```python
from build123d import *

# Parameters (mm, degrees)
SKETCH1_W           = 38.1
SKETCH1_H           = 38.1
BOSS_EXTRUDE1_DEPTH = 1.5875
SKETCH4_R           = 1.143
CUT_EXTRUDE2_DEPTH  = 7.874
SKETCH6_W           = 15.875
SKETCH6_H           = 15.875
BOSS_EXTRUDE2_DEPTH = 6.731
SKETCH7_R           = 0.889
BOSS_EXTRUDE3_DEPTH = 6.731
SKETCH8_R           = 7.747
BOSS_EXTRUDE4_DEPTH = 3.048
SKETCH9_R           = 5.969
BOSS_EXTRUDE5_DEPTH = 6.096
SKETCH10_R          = 6.985
BOSS_EXTRUDE6_DEPTH = 3.81
SKETCH11_W          = 9.906
SKETCH11_H          = 4.572
BOSS_EXTRUDE7_DEPTH = 8.255


with BuildPart() as part:
    # Sketch1 → Boss-Extrude1 (new body)
    with BuildSketch(Plane(origin=(0, 0, 0), x_dir=(1, 0, 0), z_dir=(0, 1, 0))):
        with Locations((-252.591789549, -315.673153846)):
            Rectangle(SKETCH1_W, SKETCH1_H)
    extrude(amount=BOSS_EXTRUDE1_DEPTH)

    # Sketch4 → Cut-Extrude2 (cut)
    with BuildSketch(Plane(origin=(0, 1.5875, 0), x_dir=(1, 0, 0), z_dir=(0, 1, 0))):
        with Locations((-266.561789549, -301.703153846)):
            Circle(SKETCH4_R)
        with Locations((-238.621789549, -301.703153846)):
            Circle(SKETCH4_R)
        with Locations((-266.561789549, -329.643153846)):
            Circle(SKETCH4_R)
        with Locations((-238.621789549, -329.643153846)):
            Circle(SKETCH4_R)
        with BuildLine():
            Line((-269.863789549, -312.294953846), (-269.863789549, -319.051353846))
            ThreePointArc((-269.863789549, -319.051353846), (-269.228789549, -319.686353846), (-268.593789549, -319.051353846))
            Line((-268.593789549, -319.051353846), (-268.593789549, -312.294953846))
            ThreePointArc((-268.593789549, -312.294953846), (-269.228789549, -311.659953846), (-269.863789549, -312.294953846))
        make_face()
        with BuildLine():
            Line((-259.385291519, -298.401153846), (-268.278408573, -298.401153846))
            ThreePointArc((-268.278408573, -298.401153846), (-270.0370126, -298.227930795), (-269.863789549, -299.986534822))
            Line((-269.863789549, -299.986534822), (-269.863789549, -309.246953846))
            ThreePointArc((-269.863789549, -309.246953846), (-269.228789549, -309.881953846), (-268.593789549, -309.246953846))
            Line((-268.593789549, -309.246953846), (-268.593789549, -299.986534822))
            ThreePointArc((-268.593789549, -299.986534822), (-268.420566498, -299.844376897), (-268.278408573, -299.671153846))
            Line((-268.278408573, -299.671153846), (-259.385291519, -299.671153846))
            ThreePointArc((-259.385291519, -299.671153846), (-258.750291519, -299.036153846), (-259.385291519, -298.401153846))
        make_face()
        with BuildLine():
            Line((-255.969989549, -298.401153846), (-249.213589549, -298.401153846))
            ThreePointArc((-249.213589549, -298.401153846), (-248.578589549, -299.036153846), (-249.213589549, -299.671153846))
            Line((-249.213589549, -299.671153846), (-255.969989549, -299.671153846))
            ThreePointArc((-255.969989549, -299.671153846), (-256.604989549, -299.036153846), (-255.969989549, -298.401153846))
        make_face()
        with BuildLine():
            Line((-236.589789549, -309.246953846), (-236.589789549, -299.986534822))
            ThreePointArc((-236.589789549, -299.986534822), (-236.7630126, -299.844376897), (-236.905170525, -299.671153846))
            Line((-236.905170525, -299.671153846), (-245.798287579, -299.671153846))
            ThreePointArc((-245.798287579, -299.671153846), (-246.433287579, -299.036153846), (-245.798287579, -298.401153846))
            Line((-245.798287579, -298.401153846), (-236.905170525, -298.401153846))
            ThreePointArc((-236.905170525, -298.401153846), (-235.146566498, -298.227930795), (-235.319789549, -299.986534822))
            Line((-235.319789549, -299.986534822), (-235.319789549, -309.246953846))
            ThreePointArc((-235.319789549, -309.246953846), (-235.954789549, -309.881953846), (-236.589789549, -309.246953846))
        make_face()
        with BuildLine():
            Line((-236.589789549, -312.294953846), (-236.589789549, -319.051353846))
            ThreePointArc((-236.589789549, -319.051353846), (-235.954789549, -319.686353846), (-235.319789549, -319.051353846))
            Line((-235.319789549, -319.051353846), (-235.319789549, -312.294953846))
            ThreePointArc((-235.319789549, -312.294953846), (-235.954789549, -311.659953846), (-236.589789549, -312.294953846))
        make_face()
        with BuildLine():
            Line((-245.798287579, -332.945153846), (-236.905170525, -332.945153846))
            ThreePointArc((-236.905170525, -332.945153846), (-235.146566498, -333.118376897), (-235.319789549, -331.35977287))
            Line((-235.319789549, -331.35977287), (-235.319789549, -322.099353846))
            ThreePointArc((-235.319789549, -322.099353846), (-235.954789549, -321.464353846), (-236.589789549, -322.099353846))
            Line((-236.589789549, -322.099353846), (-236.589789549, -331.35977287))
            ThreePointArc((-236.589789549, -331.35977287), (-236.7630126, -331.501930795), (-236.905170525, -331.675153846))
            Line((-236.905170525, -331.675153846), (-245.798287579, -331.675153846))
            ThreePointArc((-245.798287579, -331.675153846), (-246.433287579, -332.310153846), (-245.798287579, -332.945153846))
        make_face()
        with BuildLine():
            Line((-268.593789549, -322.099353846), (-268.593789549, -331.35977287))
            ThreePointArc((-268.593789549, -331.35977287), (-268.420566498, -331.501930795), (-268.278408573, -331.675153846))
            Line((-268.278408573, -331.675153846), (-259.385291519, -331.675153846))
            ThreePointArc((-259.385291519, -331.675153846), (-258.750291519, -332.310153846), (-259.385291519, -332.945153846))
            Line((-259.385291519, -332.945153846), (-268.278408573, -332.945153846))
            ThreePointArc((-268.278408573, -332.945153846), (-270.0370126, -333.118376897), (-269.863789549, -331.35977287))
            Line((-269.863789549, -331.35977287), (-269.863789549, -322.099353846))
            ThreePointArc((-269.863789549, -322.099353846), (-269.228789549, -321.464353846), (-268.593789549, -322.099353846))
        make_face()
        with BuildLine():
            Line((-255.969989549, -331.675153846), (-249.213589549, -331.675153846))
            ThreePointArc((-249.213589549, -331.675153846), (-248.578589549, -332.310153846), (-249.213589549, -332.945153846))
            Line((-249.213589549, -332.945153846), (-255.969989549, -332.945153846))
            ThreePointArc((-255.969989549, -332.945153846), (-256.604989549, -332.310153846), (-255.969989549, -331.675153846))
        make_face()
    extrude(amount=-CUT_EXTRUDE2_DEPTH, mode=Mode.SUBTRACT)

    # Sketch6 → Boss-Extrude2 (add)
    with BuildSketch(Plane(origin=(0, 1.5875, 0), x_dir=(1, 0, 0), z_dir=(0, 1, 0))):
        with Locations((-252.591789549, -315.673153846)):
            Rectangle(SKETCH6_W, SKETCH6_H)
    extrude(amount=BOSS_EXTRUDE2_DEPTH)

    # Sketch7 → Boss-Extrude3 (add)
    with BuildSketch(Plane(origin=(0, 1.5875, 0), x_dir=(1, 0, 0), z_dir=(0, 1, 0))):
        with BuildLine():
            Line((-242.622289549, -313.641153846), (-244.654289549, -313.641153846))
            Line((-244.654289549, -313.641153846), (-244.654289549, -317.705153846))
            Line((-244.654289549, -317.705153846), (-242.622289549, -317.705153846))
            ThreePointArc((-242.622289549, -317.705153846), (-240.590289549, -315.673153846), (-242.622289549, -313.641153846))
        make_face()
        with Locations((-242.622289549, -315.673153846)):
            Circle(SKETCH7_R, mode=Mode.SUBTRACT)
        with BuildLine():
            Line((-262.561289549, -317.705153846), (-260.529289549, -317.705153846))
            Line((-260.529289549, -317.705153846), (-260.529289549, -313.641153846))
            Line((-260.529289549, -313.641153846), (-262.561289549, -313.641153846))
            ThreePointArc((-262.561289549, -313.641153846), (-264.593289549, -315.673153846), (-262.561289549, -317.705153846))
        make_face()
        with Locations((-262.561289549, -315.673153846)):
            Circle(SKETCH7_R, mode=Mode.SUBTRACT)
    extrude(amount=BOSS_EXTRUDE3_DEPTH)

    # Sketch8 → Boss-Extrude4 (add)
    with BuildSketch(Plane(origin=(0, 8.3185, 0), x_dir=(1, 0, 0), z_dir=(0, 1, 0))):
        with Locations((-252.436354268, -315.828589127)):
            Circle(SKETCH8_R)
    extrude(amount=BOSS_EXTRUDE4_DEPTH)

    # Sketch9 → Boss-Extrude5 (add)
    with BuildSketch(Plane(origin=(0, 11.3665, 0), x_dir=(1, 0, 0), z_dir=(0, 1, 0))):
        with Locations((-252.465375739, -315.583143422)):
            Circle(SKETCH9_R)
    extrude(amount=BOSS_EXTRUDE5_DEPTH)

    # Sketch10 → Boss-Extrude6 (add)
    with BuildSketch(Plane(origin=(0, 17.4625, 0), x_dir=(1, 0, 0), z_dir=(0, 1, 0))):
        with Locations((-252.465375739, -315.583143422)):
            Circle(SKETCH10_R)
    extrude(amount=BOSS_EXTRUDE6_DEPTH)

    # Sketch11 → Boss-Extrude7 (add)
    with BuildSketch(Plane.XZ):
        with Locations((-256.737392156, 301.957153846)):
            Rectangle(SKETCH11_W, SKETCH11_H)
    extrude(amount=BOSS_EXTRUDE7_DEPTH)


solid = part.part
```
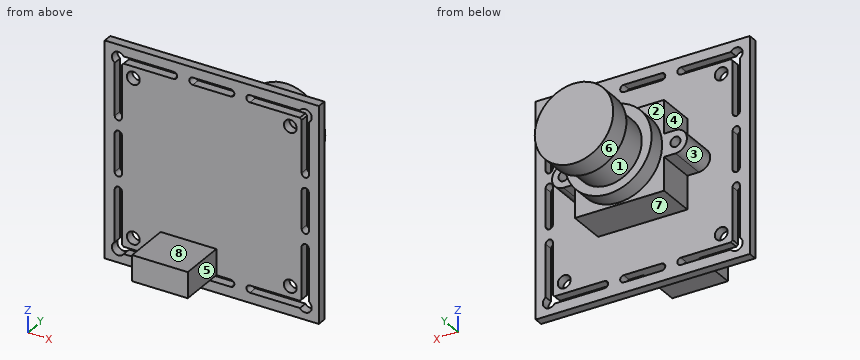
Could you check a few things on this model? Use its own coordinates, in mm. Face numbers are marked on the shaded views. A direction names the side the tool comes from. Round coordinates to 2 decimals unless told otherwise and drop trailing zeros. Loops run counter-clockwise (first coordinate to the right, second up) from the corner with the lowest first, then second, coordinate; pieces in that order, holes last. Notation, with made-up numbers: (23.5, 86) -> (55.5, 86) arc R31 ccw to (55.5, 111) -> close; hole circle Ø8 at (-7, 62.5). An arc over 180 degrees is marked (long way). One line per question, with ' | ' between items.
(1) Thinking about a two-plate mould opening in Y: for the marked faces 1, 2 and 3, which applies, released by +Y, released by -Y, zero draft, split by the parting line, or undercut?
Model answer:
face 1: undercut | face 2: released by +Y | face 3: zero draft
(2) If we section it at A-A on x = -238.5: List the corners of the cut face in (y, z) for me.
Model answer:
outline: (0, 296.62) -> (1.59, 296.62) -> (1.59, 298.4) -> (0, 298.4) -> close; (0, 299.67) -> (1.59, 299.67) -> (1.59, 300.57) -> (0, 300.57) -> close; (0, 302.84) -> (1.59, 302.84) -> (1.59, 328.51) -> (0, 328.51) -> close; (0, 330.78) -> (1.59, 330.78) -> (1.59, 331.68) -> (0, 331.68) -> close; (0, 332.95) -> (1.59, 332.95) -> (1.59, 334.72) -> (0, 334.72) -> close
(3) If we section it at C-C on y = 7.75: List the corners of the cut face in (x, z) for me, and give its area (3 significant figures).
Model answer:
outline: (-262.56, 313.64) -> (-260.53, 313.64) -> (-260.53, 307.74) -> (-244.65, 307.74) -> (-244.65, 313.64) -> (-242.62, 313.64) arc R2.03 ccw to (-242.62, 317.71) -> (-244.65, 317.71) -> (-244.65, 323.61) -> (-260.53, 323.61) -> (-260.53, 317.71) -> (-262.56, 317.71) arc R2.03 ccw to start; hole circle Ø1.78 at (-262.56, 315.67); hole circle Ø1.78 at (-242.62, 315.67) | area: 277 mm^2
(4) If we section it at D-D on x = -250: List the corners of the cut face in (y, z) for me.
Model answer:
outline: (0, 296.62) -> (1.59, 296.62) -> (1.59, 298.4) -> (0, 298.4) -> close; (0, 299.67) -> (1.59, 299.67) -> (1.59, 307.74) -> (8.32, 307.74) -> (8.32, 308.47) -> (11.37, 308.47) -> (11.37, 310.15) -> (17.46, 310.15) -> (17.46, 309.05) -> (21.27, 309.05) -> (21.27, 322.12) -> (17.46, 322.12) -> (17.46, 321.02) -> (11.37, 321.02) -> (11.37, 323.18) -> (8.32, 323.18) -> (8.32, 323.61) -> (1.59, 323.61) -> (1.59, 331.68) -> (0, 331.68) -> close; (0, 332.95) -> (1.59, 332.95) -> (1.59, 334.72) -> (0, 334.72) -> close
(5) If I drill on probe 1 along X at (y, z) = (0.5, 327.5); probe 2 along Y at (x, z) = (-257, 311.5); probe 3 along X at (y, z) = (2.25, 321), over which ranges is the centre line in solid material (lowest first)?
Model answer:
probe 1: x = -271.64 to -269.86, -268.59 to -236.59, -235.32 to -233.54 | probe 2: y = 0 to 11.37, 17.46 to 21.27 | probe 3: x = -260.53 to -244.65
(6) For the marked faces 4, 5, 6, 7 and 8, which set-ups out of +Z, -Z, +X, -X, +Y, -Y let a thin tool reach every point of the face, with its end or its side?
Model answer:
face 4: +Z, -X, +Y | face 5: +Z, -Z, +X, -Y | face 6: +Y | face 7: -Z, +X, -X, +Y | face 8: +Z, +X, -X, -Y
(7) If we section it at B-B on z = 325.5: List the corners of the cut face in (x, y) for me.
Model answer:
outline: (-271.64, 0) -> (-269.86, 0) -> (-269.86, 1.59) -> (-271.64, 1.59) -> close; (-268.59, 0) -> (-236.59, 0) -> (-236.59, 1.59) -> (-268.59, 1.59) -> close; (-235.32, 0) -> (-233.54, 0) -> (-233.54, 1.59) -> (-235.32, 1.59) -> close
(8) For pin 1 Ø3 at (x, z) = (-242.62, 315.67) entering from -Y; pin 2 Ø2 at (x, y) = (-250.5, 6) entering from -Z; pin 3 Ø5 at (y, z) = (-5.5, 302.5) entering from -X, each with a flat end and sliding along its axis, tell me the tip position at first contact or that it passes through.
Model answer:
pin 1: stops at y = 0 | pin 2: stops at z = 307.74 | pin 3: stops at x = -261.69
